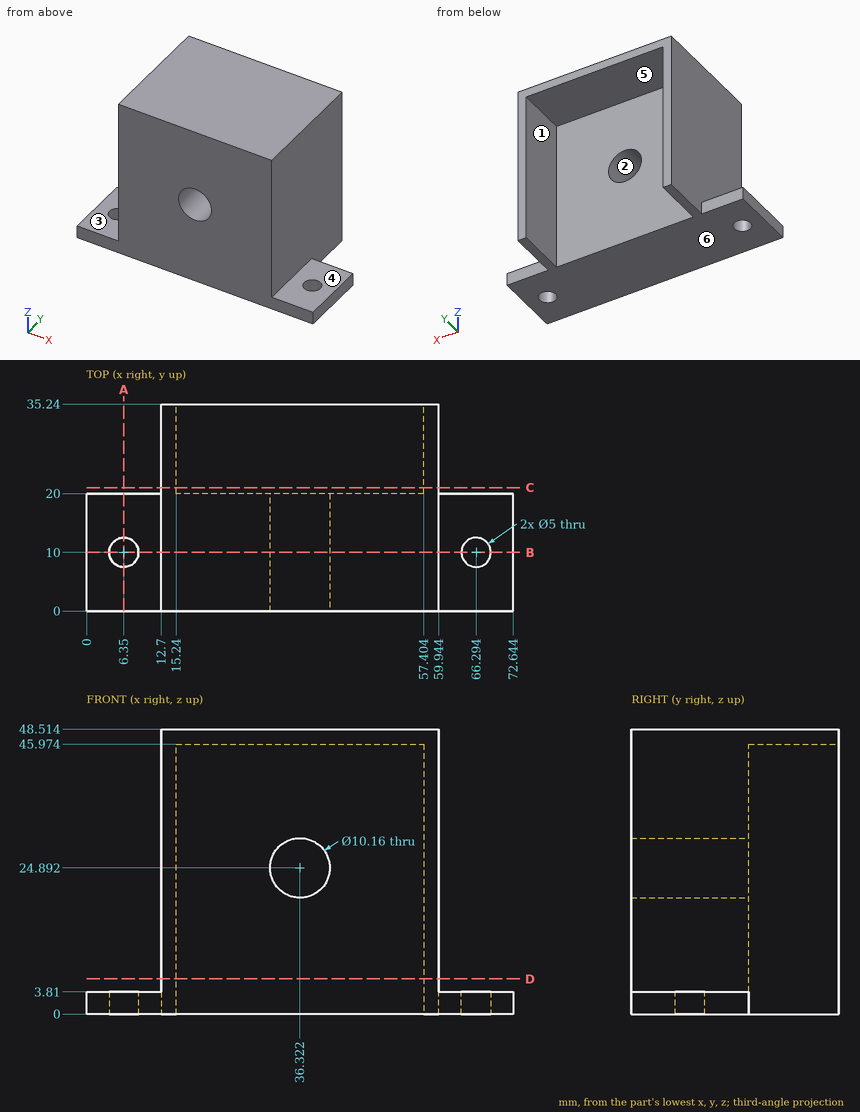
The drawing under review shows one solid part. Ordinate dimensions are in mm from its lowest x, y, z. A direction names the side the tool comes from. Give positions to 0.01 mm unless a question says otherwise; leave off trailing zeros. Write each loop counter-clockwise with the first axis right and the second up, starting at its lowest first coordinate (ties: lowest second). Pieces come first, ordered by that corner, then holes. Notation, with made-up numbers: (75.5, 89) - (103.5, 89) arc R22 cw to (103.5, 113) - close; hole circle Ø9 at (12.5, -8.5). An arc over 180 degrees is marked (long way). Answer in a Markdown table with one row per item. Add a question column.
1. We need section B-B on y = 10. Write out the cut boundary in (x, z), then the cut area to 3 significant figures.
2. Tool access review of the marked faces 4, 5 and 6: name each direction out of +Z, -Z, +X, -X, +Y, -Y from which nothing blocks a thin tool from reaching the whole face with its end or side.
3. We need section A-A on x = 6.35. Write out the cut boundary in (y, z), then the cut area to 4 significant figures.
4. We need section D-D on z = 6. Write out the cut boundary in (x, y).
5. Insertion check: P1, Ø8, axis at x = 66.294, y = 10, coming from the -Z side; P2, Ø4, axis at y = 4, z = 33, coming from the +X side; P3, Ø4, axis at x = 7, z = 2.5, coming from the +Y side; P4, Ø12, axis at x = 39.5, y = 30, coming from the -Z side. Each pin has a flat end and moves straight along its axis. Give the tip position at first contact, or say it passes through.
6. Wall thickness on line 1 along X through (y, z) = (22, 18.5); line 2 along Y through (x, z) = (18.5, 4); line 3 along X through (y, z) = (10.5, 45): over which ranges is each line inside the solid? List them lowest first. Write a range as [from, to].
7. We need section C-C on y = 21. Write out the cut boundary in (x, z).
8. Draft analysis for pull direction X (two halves, no side actions). For the marked faces 1, 2 and 3, state which applies: +X half, -X half, draft (parallel to the pull), parting line (faces both ways), or undercut.
Ans:
| question | item | result |
|---|---|---|
| 1 | outline | (0, 0) - (3.85, 0) - (3.85, 3.81) - (0, 3.81) - close; (8.85, 0) - (63.79, 0) - (63.79, 3.81) - (59.94, 3.81) - (59.94, 48.51) - (12.7, 48.51) - (12.7, 3.81) - (8.85, 3.81) - close; (68.79, 0) - (72.64, 0) - (72.64, 3.81) - (68.79, 3.81) - close; hole circle Ø10.16 at (36.32, 24.89) |
| 1 | area | 2,270 mm^2 |
| 2 | face 4 | +Z, +X, +Y, -Y |
| 2 | face 5 | -Z, +Y |
| 2 | face 6 | -Z, +X, -X, +Y, -Y |
| 3 | outline | (0, 0) - (7.5, 0) - (7.5, 3.81) - (0, 3.81) - close; (12.5, 0) - (20, 0) - (20, 3.81) - (12.5, 3.81) - close |
| 3 | area | 57.15 mm^2 |
| 4 | outline | (12.7, 0) - (59.94, 0) - (59.94, 35.24) - (57.4, 35.24) - (57.4, 20) - (15.24, 20) - (15.24, 35.24) - (12.7, 35.24) - close |
| 5 | P1 | stops at z = 0 |
| 5 | P2 | stops at x = 59.94 |
| 5 | P3 | stops at y = 20 |
| 5 | P4 | stops at z = 45.97 |
| 6 | line 1 | x = [12.7, 15.24], [57.4, 59.94] |
| 6 | line 2 | y = [0, 20] |
| 6 | line 3 | x = [12.7, 59.94] |
| 7 | outline | (12.7, 0) - (15.24, 0) - (15.24, 45.97) - (57.4, 45.97) - (57.4, 0) - (59.94, 0) - (59.94, 48.51) - (12.7, 48.51) - close |
| 8 | face 1 | undercut |
| 8 | face 2 | undercut |
| 8 | face 3 | draft |
